from build123d import *

# Parameters (mm, degrees)
PAD_DEPTH       = 4.75
PAD001_DEPTH    = 4.75
FILLET_R        = 4
CHAMFER_SIZE    = 2
SKETCH002_R     = 3.95
POCKET_DEPTH    = 2.75
SKETCH003_R     = 3.95
POCKET001_DEPTH = 2.75
SKETCH004_R     = 2.15
POCKET002_DEPTH = 2.001
SKETCH005_R     = 2.15
POCKET003_DEPTH = 2.001


with BuildPart() as part:
    # Sketch → Pad (new body)
    with BuildSketch(Plane.XY):
        with BuildLine():
            Line((-9.75, 8), (0, 8))
            Line((0, 8), (0, -8))
            Line((0, -8), (-9.749974, -8))
            ThreePointArc((-9.75, 8), (-17.749974, -1.3e-05), (-9.749974, -8))
        make_face()
    extrude(amount=PAD_DEPTH)

    # Sketch001 → Pad001 (new body)
    with BuildSketch(Plane.YZ):
        with BuildLine():
            Line((-8, 9.75), (-8, 0))
            Line((-8, 0), (8, 0))
            Line((8, 0), (8, 9.749968))
            ThreePointArc((8, 9.749968), (1.6e-05, 17.749968), (-8, 9.75))
        make_face()
    extrude(amount=-PAD001_DEPTH)

    # Fillet
    fillet_edges = [part.edges().sort_by_distance(p)[0] for p in [
        (-4.75, 0, 4.75),
    ]]
    fillet(fillet_edges, radius=FILLET_R)

    # Chamfer
    chamfer_edges = [part.edges().sort_by_distance(p)[0] for p in [
        (-17.749974, -1.3e-05, 4.75),
    ]]
    chamfer(chamfer_edges, length=CHAMFER_SIZE)

    # Sketch002 → Pocket (cut, symmetric)
    with BuildSketch(Plane.XY.offset(4.75)):
        with Locations((-9.749974, 0)):
            Circle(SKETCH002_R)
    extrude(amount=POCKET_DEPTH, both=True, mode=Mode.SUBTRACT)

    # Sketch003 → Pocket001 (cut, symmetric)
    with BuildSketch(Plane(origin=(-4.75, 0, 0), x_dir=(0, -1, 0), z_dir=(-1, 0, 0))):
        with Locations((0, 9.749968)):
            Circle(SKETCH003_R)
    extrude(amount=POCKET001_DEPTH, both=True, mode=Mode.SUBTRACT)

    # Sketch004 → Pocket002 (cut, through all)
    with BuildSketch(Plane(origin=(-2, 0, 0), x_dir=(0, -1, 0), z_dir=(-1, 0, 0))):
        with Locations((0, 9.749968)):
            Circle(SKETCH004_R)
    extrude(amount=-POCKET002_DEPTH, mode=Mode.SUBTRACT)

    # Sketch005 → Pocket003 (cut, through all)
    with BuildSketch(Plane.XY.offset(2)):
        with Locations((-9.749974, 0)):
            Circle(SKETCH005_R)
    extrude(amount=-POCKET003_DEPTH, mode=Mode.SUBTRACT)


solid = part.part
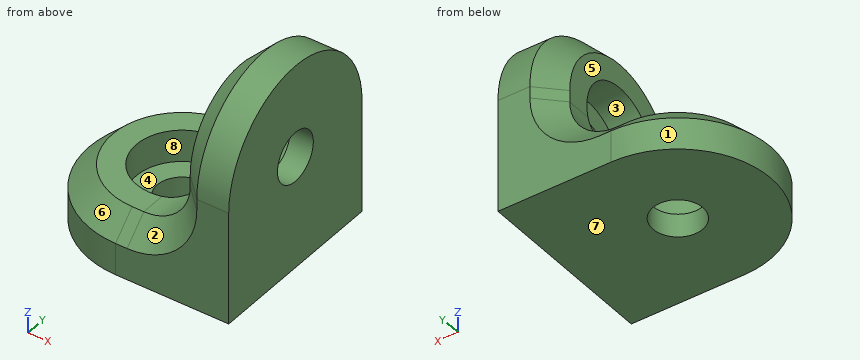
Verification items for the finished model (mm, model axes). Face numbers are marked on the shaded views. A direction names the side the tool comes from. Round coordinates to 2 decimals unless told otherwise and drop trailing zeros. Write each loop counter-clockwise with the first axis right and the second up, starting at its lowest first coordinate (ties: lowest second). Pieces come first, ordered by that corner, then holes.
(1) Access from +Z, -Z, +X, -X, +Y, -Y to the whole of each face (thin tool, end or side, straight path). Record for the marked faces 1, 2, 3, 4 and 5.
Returned:
face 1: +Z, -Z, -X
face 2: +Z, -X, -Y
face 3: -X
face 4: +Z
face 5: +Z, -X, +Y, -Y
(2) Section check A-A (y = 0). Enter the section's corners in (x, z), plus the area to 3 significant figures.
Returned:
outline: (-17.75, 0) - (-11.9, 0) - (-11.9, 2) - (-13.7, 2) - (-13.7, 4.75) - (-15.75, 4.75) - (-17.75, 2.75) - close; (-7.6, 0) - (0, 0) - (0, 7.6) - (-2, 7.6) - (-2, 5.8) - (-5.8, 5.8) - (-5.8, 2) - (-7.6, 2) - close; (-4.75, 13.7) - (-2, 13.7) - (-2, 11.9) - (0, 11.9) - (0, 17.75) - (-2.75, 17.75) - (-4.75, 15.75) - close
area: 82.5 mm2
(3) Material ranges on line 1 (Z direction, x = -1.2, y = 0); line 2 (X direction, y = 4.5, z = 9.75); line 3 (Y direction, x = -3, z = 10.25), recorded low to high.
Returned:
line 1: z = 0 to 7.6, 11.9 to 17.75
line 2: x = -4.75 to 0
line 3: y = -7.73 to -3.92, 3.92 to 7.73
(4) Section check B-B (z = 1.75). Enter the section's corners in (x, y).
Returned:
outline: (-9.75, -8) - (0, -8) - (0, 8) - (-9.75, 8) arc R8 ccw to start; hole circle Ø4.3 at (-9.75, 0)
(5) Mould release check, pull along Y, two halves, no side actions. Record for the marked faces 6, 7 and 8: pulls with the +Y half, pulls with the -Y half, needs draft (parallel to the pull), parting line crosses it, or undercut.
Returned:
face 6: parting line crosses it
face 7: needs draft
face 8: undercut
(6) Depth check by flat-ended pin: pin 1 Ø7.5 at (y, z) = (0, 13.5) entering from -X; pin 2 Ø4 at (y, z) = (4, 2) entering from -X; pin 3 Ø3.5 at (x, y) = (-9.75, 0) entering from +Z; pin 4 Ø4 at (y, z) = (5.5, 6) entering from -X. Enter the tip coordinate at first touch or a pass-through.
Returned:
pin 1: stops at x = -4.75
pin 2: stops at x = -17.5
pin 3: passes through
pin 4: stops at x = -14.43
